CAD build for the part. Positions are in the model's coordinates, mm. A direction names the side the tool comes from. Coordinates: 2 decimals unless noted, no trailing zeros. Loops run counter-clockwise (first coordinate to the right, second up) from the corner with the lowest first, then second, coordinate; pieces in that order, holes last. Notation, with made-up numbers: (20, 22) - (57, 22) arc R15 ccw to (57, 43) - close; hole circle Ø8 at (-10, 23.25). An arc over 180 degrees is marked (long way). Put each result on its own line as item: value.
```python
from build123d import *

# Parameters (mm, degrees)
CHANFRO1_SIZE = 1
CHANFRO2_SIZE = 1


with BuildPart() as part:
    # Esboço1 → Revolução1 (revolve)
    with BuildSketch(Plane(origin=(0, 0, 0), x_dir=(0, 0, -1), z_dir=(1, 0, 0))):
        Polygon((18, 18.768101913), (10.5, 18.768101913), (10.5, 21.768101913), (12, 21.768101913), (12, 31.768101913), (7, 31.768101913), (7, -7.231898087), (8.495318128, -7.231898087), (18.5883066, 17.749124991), align=None)
    revolve(axis=Axis((0, 0, 0), (0, 1, 0)))

    # Chanfro1
    chanfro1_edges = [part.edges().sort_by_distance(p)[0] for p in [
        (0, 31.768101913, 12),
    ]]
    chamfer(chanfro1_edges, length=CHANFRO1_SIZE)

    # Chanfro2
    chanfro2_edges = [part.edges().sort_by_distance(p)[0] for p in [
        (0, 21.768101913, 12),
    ]]
    chamfer(chanfro2_edges, length=CHANFRO2_SIZE)


solid = part.part
```
Q1. Slice it at B-B, the plane z = 0. Give the cut face in (x, y), then the cut area to 3 significant figures.
Determined:
outline: (-18.59, 17.75) - (-8.5, -7.23) - (-7, -7.23) - (-7, 31.77) - (-11, 31.77) - (-12, 30.77) - (-12, 22.77) - (-11, 21.77) - (-10.5, 21.77) - (-10.5, 18.77) - (-18, 18.77) - close; (7, -7.23) - (8.5, -7.23) - (18.59, 17.75) - (18, 18.77) - (10.5, 18.77) - (10.5, 21.77) - (11, 21.77) - (12, 22.77) - (12, 30.77) - (11, 31.77) - (7, 31.77) - close
area: 469 mm2
Q2. Slice it at A-A, the plane x = 0. Give the cut face in (y, z).
Determined:
outline: (-7.23, -8.5) - (17.75, -18.59) - (18.77, -18) - (18.77, -10.5) - (21.77, -10.5) - (21.77, -11) - (22.77, -12) - (30.77, -12) - (31.77, -11) - (31.77, -7) - (-7.23, -7) - close; (-7.23, 7) - (31.77, 7) - (31.77, 11) - (30.77, 12) - (22.77, 12) - (21.77, 11) - (21.77, 10.5) - (18.77, 10.5) - (18.77, 18) - (17.75, 18.59) - (-7.23, 8.5) - close
Q3. Tool access for faces 4 (the flat face through (-0.2, 31.768, -7.2)), 5 (the flat face through (4, 21.768, 10)): list every direction of +Z, -Z, +X, -X, +Y, -Y with a clear straight run to the whole face (end or side of a thin tool).
Determined:
face 4: +Z, -Z, +X, -X, +Y
face 5: none
Q4. Mould opens along Y. For faces 1 (the cylindrical face through (-0.53, 26.82, 11.99)), 2 (the cylindrical face through (-3.2, 20.3, -10)), 3 (the conical face through (11.1, -0.1, 2.5)) say: +Y half, -Y half, draft (parallel to the pull), parting line (faces both ways), or undercut.
Determined:
face 1: draft
face 2: undercut
face 3: -Y half
Q5. Pin check, flat tips, straight feed: pin 1 Ø4 at (y, z) = (4, 5.5) entering from +X; pin 2 Ø1.5 at (y, z) = (26.5, -6.5) entering from +X; pin 3 Ø6 at (x, y) = (12.5, 15.5) entering from +Z. Stop position of each tip, or through.
Determined:
pin 1: x = 12.99
pin 2: x = 10.53
pin 3: z = 15.39
Q6. Slice it at C-C, the plane y = 26. Give the cut face in (x, z), then the cut area to 3 significant figures.
Determined:
outline: circle Ø24 at (0, 0); hole circle Ø14 at (0, 0)
area: 298 mm2
Q7. Slice it at D-D, the plane y = -4.5. Give the cut face in (x, z).
Determined:
outline: circle Ø19.2 at (0, 0); hole circle Ø14 at (0, 0)
Q8. Wall check: L1, parallel to X at y = 23.5, z = 0; L2, parallel to X at y = 14, z = 0; L3, parallel to Z at x = 0, y = 15. Give the ranges that are in metal, low to high. Write a range as from..to.
Determined:
L1: -12..-7, 7..12
L2: -17.07..-7, 7..17.07
L3: -17.48..-7, 7..17.48
